```python
from build123d import *

# Parameters (mm, degrees)
SKETCH_1_W        = 50
SKETCH_1_H        = 50
EXTRUDE_1_DEPTH   = 10
HOLE_WIZARD_339_D = 24
HOLE_WIZARD_2_D   = 3.2
HOLE_WIZARD_3_D   = 10


with BuildPart() as part:
    # 草图1 → 凸台-拉伸1 (new body)
    with BuildSketch(Plane.XY):
        Rectangle(SKETCH_1_W, SKETCH_1_H)
    extrude(amount=EXTRUDE_1_DEPTH)

    # Hole Wizard 339 (through all)
    with Locations(Plane.XY.offset(10)):
        with Locations((0, 0)):
            Hole(HOLE_WIZARD_339_D / 2)

    # 孔2 (through all)
    with Locations(Plane.XY.offset(10)):
        with Locations((0, 18.5), (18.5, 0), (0, -18.5), (-18.5, 0)):
            Hole(HOLE_WIZARD_2_D / 2)

    # 孔3 (through all)
    with Locations(Plane.XY.offset(10)):
        with Locations((-15.5, 15.5), (15.5, 15.5), (15.5, -15.5), (-15.5, -15.5)):
            Hole(HOLE_WIZARD_3_D / 2)


solid = part.part
```
CAD build for the part. Positions are in the model's coordinates, mm. Coordinates: 2 decimals unless noted, no trailing zeros. Write each loop counter-clockwise with the first axis right and the second up, starting at its lowest first coordinate (ties: lowest second). Pieces come first, ordered by that corner, then holes.
(1) Cut at C-C, the plane x = 0. List the corners of the cut face in (y, z).
(2) Cut at D-D, the plane z = 9.25. Count the separate pieces of the cut face and the enclosed holes in it, and give its area (3 significant figures).
(3) Two-plate mould, pull along Y, no slides. Class faces 1 (the face through (0, -25, 5)), 2 (the face through (25, 0, 5)), 3 (the face through (-17.807, 11.064, 4.93)), 4 (the face through (0, 25, 5)): +Y half, -Y half, draft (parallel to the pull), parting line (faces both ways), or undercut.
(4) Cut at A-A, the plane x = -15.5. List the corners of the cut face in (y, z), and give its area (3 significant figures).
(5) Drill centre lines: probe 1 along Y at (x, z) = (-15.5, 7.5); probe 2 along Y at (x, z) = (0, 3.25); probe 3 along Y at (x, z) = (-18, 5). Where is each one in solid material? Low to high.
(6) Flat gauge pin, fed straight in: pin 1 (5 mm diameter, centred on x = 16.5, y = 1, fed in from -Z). Where does the tip first touch, or does it go through?
Geometry says:
1. outline: (-25, 0) - (-20.1, 0) - (-20.1, 10) - (-25, 10) - close; (-16.9, 0) - (-12, 0) - (-12, 10) - (-16.9, 10) - close; (12, 0) - (16.9, 0) - (16.9, 10) - (12, 10) - close; (20.1, 0) - (25, 0) - (25, 10) - (20.1, 10) - close
2. separate pieces: 1
2. enclosed holes: 9
2. area: 1,700 mm2
3. face 1: -Y half
3. face 2: draft
3. face 3: undercut
3. face 4: +Y half
4. outline: (-25, 0) - (-20.5, 0) - (-20.5, 10) - (-25, 10) - close; (-10.5, 0) - (10.5, 0) - (10.5, 10) - (-10.5, 10) - close; (20.5, 0) - (25, 0) - (25, 10) - (20.5, 10) - close
4. area: 300 mm2
5. probe 1: y = -25 to -20.5, -10.5 to 10.5, 20.5 to 25
5. probe 2: y = -25 to -20.1, -16.9 to -12, 12 to 16.9, 20.1 to 25
5. probe 3: y = -25 to -19.83, -11.17 to -1.52, 1.52 to 11.17, 19.83 to 25
6. pin 1: stops at z = 0
